Print and shaded views of the part. All mm, measured from the part's lowest x, y and z. A direction names the side the tool comes from. Round coordinates to 2 decimals unless told otherwise and drop trailing zeros. Loops run counter-clockwise (first coordinate to the right, second up) from the corner with the lowest first, then second, coordinate; pieces in that order, holes last. Notation, with made-up numbers: (33, 17) - (67, 17) arc R16 cw to (67, 29) - close; hole circle Ø9 at (-3.75, 25.5). An arc over 180 degrees is marked (long way). Put each result on its own line as item: value. Start each with the question number.
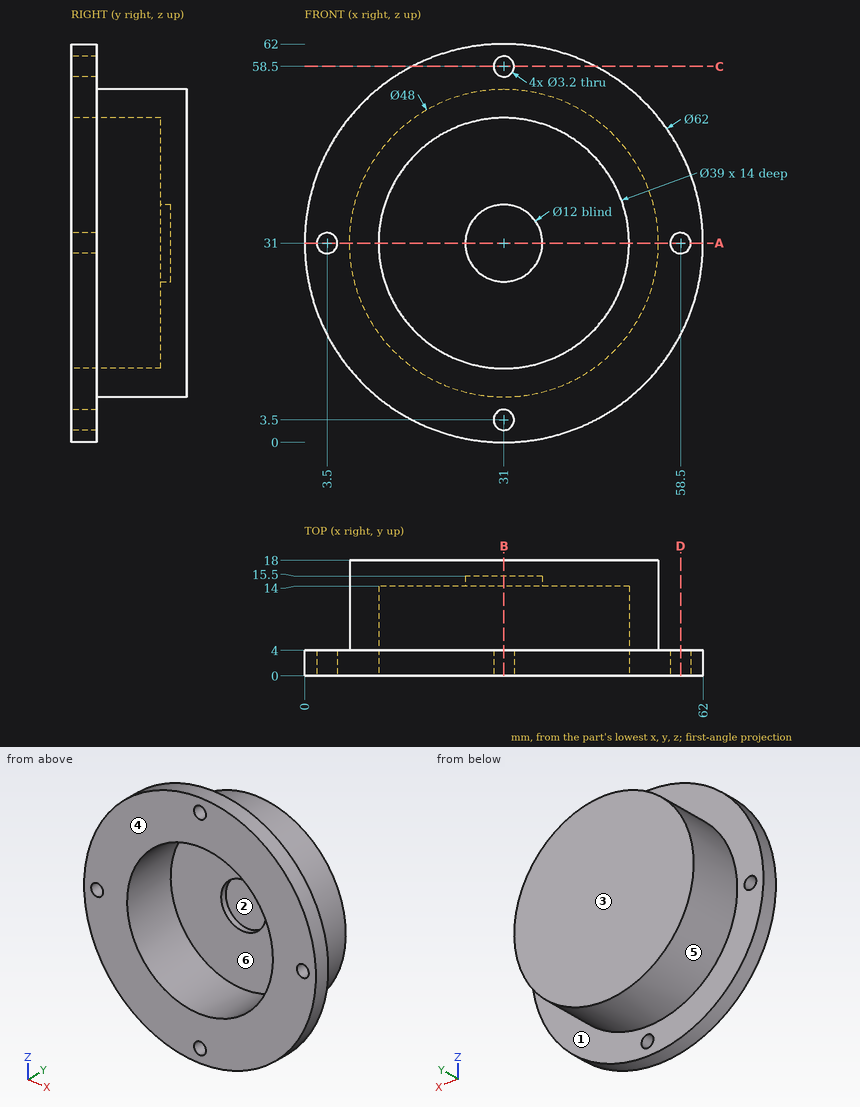
Item 1: Which spindle directions (+Z, -Z, +X, -X, +Y, -Y) get a long thin tool onto all of the face, cutting with end or side? Do the marked faces 1, 2 and 3. Say none if no direction does.
Item 2: Slice it at B-B (x = 31). Give the cut face in (y, z).
Item 3: Slice it at A-A (z = 31). Give the cut face in (x, y), plus the area to 3 significant figures.
Item 4: Drop flat-ended pins along their axis: pin 1 Ø6 at (y, z) = (14.5, 9.5) entering from +X; pin 2 Ø8 at (x, z) = (27, 45) entering from -Y; pin 3 Ø4 at (y, z) = (10, 34) entering from -X. Give the stop position or say it passes through.
Item 5: Slice it at C-C (z = 58.5). Give the cut face in (x, y), plus the area to 3 significant figures.
Item 6: Two-plate mould, pull along Z, no slides. Class the marked faces 4, 5 and 6: pulls with the +Z half, pulls with the -Z half, needs draft (parallel to the pull), parting line crosses it, or undercut.
Item 7: Slice it at D-D (x = 58.5). Give the cut face in (y, z), plus the area to 3 significant figures.
Item 8: Drill centre lines: probe 1 along X at (y, z) = (14.4, 31); probe 2 along X at (y, z) = (1.55, 31); probe 3 along X at (y, z) = (6.5, 31). Where is each one in solid material? Low to high. Write a range as [from, to].
Computed values:
1. face 1: +Y
1. face 2: -Y
1. face 3: +Z, -Z, +X, -X, +Y
2. outline: (0, 0) - (4, 0) - (4, 1.9) - (0, 1.9) - close; (0, 5.1) - (4, 5.1) - (4, 7) - (18, 7) - (18, 55) - (4, 55) - (4, 56.9) - (0, 56.9) - (0, 50.5) - (14, 50.5) - (14, 37) - (15.5, 37) - (15.5, 25) - (14, 25) - (14, 11.5) - (0, 11.5) - close; (0, 60.1) - (4, 60.1) - (4, 62) - (0, 62) - close
3. outline: (0, 0) - (1.9, 0) - (1.9, 4) - (0, 4) - close; (5.1, 0) - (11.5, 0) - (11.5, 14) - (25, 14) - (25, 15.5) - (37, 15.5) - (37, 14) - (50.5, 14) - (50.5, 0) - (56.9, 0) - (56.9, 4) - (55, 4) - (55, 18) - (7, 18) - (7, 4) - (5.1, 4) - close; (60.1, 0) - (62, 0) - (62, 4) - (60.1, 4) - close
3. area: 330 mm^2
4. pin 1: stops at x = 46.29
4. pin 2: stops at y = 14
4. pin 3: stops at x = 7.02
5. outline: (16.69, 0) - (29.4, 0) - (29.4, 4) - (16.69, 4) - close; (32.6, 0) - (45.31, 0) - (45.31, 4) - (32.6, 4) - close
5. area: 102 mm^2
6. face 4: needs draft
6. face 5: parting line crosses it
6. face 6: undercut
7. outline: (0, 16.69) - (4, 16.69) - (4, 29.4) - (0, 29.4) - close; (0, 32.6) - (4, 32.6) - (4, 45.31) - (0, 45.31) - close
7. area: 102 mm^2
8. probe 1: x = [7, 25], [37, 55]
8. probe 2: x = [0, 1.9], [5.1, 11.5], [50.5, 56.9], [60.1, 62]
8. probe 3: x = [7, 11.5], [50.5, 55]
